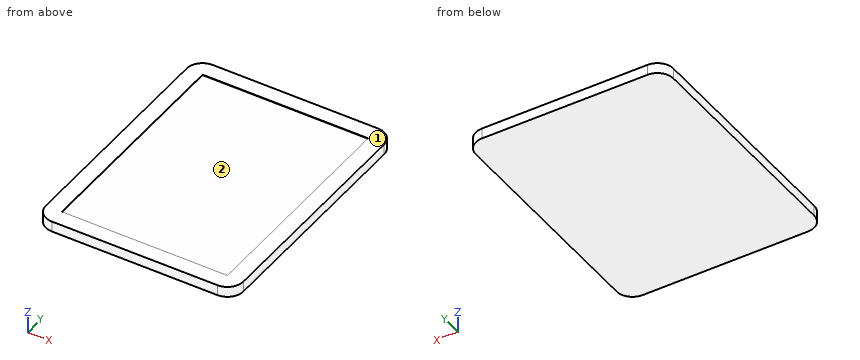
Autodesk Inventor part; units mm, degrees
ref_plane "YZ Plane" through (0, 0, 0) normal (1, 0, 0) x (0, 1, 0)
ref_plane "XZ Plane" through (0, 0, 0) normal (0, 1, 0) x (-1, 0, 0)
ref_plane "XY Plane" through (0, 0, 0) normal (0, 0, 1) x (1, 0, 0)
sketch "Skizze1" plane through (0, 0, 0) normal (0, 0, 1) x (1, 0, 0)
  line L0 (-93, 120.5) -> (93, 120.5)
  line L1 (93, 120.5) -> (93, -120.5)
  line L2 (93, -120.5) -> (-93, -120.5)
  line L3 (-93, -120.5) -> (-93, 120.5)
  line L4 (-130.2, 0) -> (130.2, 0)
  line L5 (0, -168.7) -> (0, 168.7)
  point P0 (0, 0)
  dimension "d0" = 241
  dimension "d1" = 186
extrude "Extrusion1" add sketch "Skizze1" along normal blind 10
sketch "Skizze3" plane through (0, 0, 10) normal (0, 0, 1) x (1, 0, 0)
  line L0 (93, 120.5) -> (93, -120.5)
  line L1 (-93, 120.5) -> (93, 120.5)
  line L2 (-93, -120.5) -> (-93, 120.5)
  line L3 (93, -120.5) -> (-93, -120.5)
  line L4 (78, 105.5) -> (78, -105.5)
  line L5 (78, -105.5) -> (-78, -105.5)
  line L6 (-78, -105.5) -> (-78, 105.5)
  line L7 (-78, 105.5) -> (78, 105.5)
  point P0 (0, 0)
  dimension "d5" = 15
extrude "Extrusion2" cut sketch "Skizze3" against normal blind 0.5 contours L4 L5 L6 L7
fillet "Rundung2" radius 15 4 edges at (-93, -120.5, 5) (93, -120.5, 5) (93, 120.5, 5) (-93, 120.5, 5)
properties part number "tablet"
The model under review builds one solid part; all positions refer to its coordinate system, in mm. Face numbers are marked on the shaded views. A direction names the side the tool comes from. Give positions to 0.01 mm unless a question says otherwise; leave off trailing zeros. Write each loop counter-clockwise with the first axis right and the second up, starting at its lowest first coordinate (ties: lowest second). Pieces come first, ordered by that corner, then holes. Notation, with made-up numbers: M 56,44.5 L 86,44.5 A11 cw 86,52.5 Z; hole C 37.25,-9.75 d9. An arc over 180 degrees is marked long. Answer in a Markdown table with one row per item.
Item 1: For P1, Ø5, axis at x = 5.5, y = 26.5, coming from the -Z side; P2, Ø10, axis at x = 49, y = 7, coming from the +Z side, all flat-tipped, find the tip position at first contact; note any pin that passes through.
Check sheet entries:
| item | result |
|---|---|
| P1 | z = 0 |
| P2 | z = 9.5 |
Item 2: Add section B-B on y = -23. Give the boundary of the cut face in (x, z).
Check sheet entries:
| item | result |
|---|---|
| outline | M -93,0 L 93,0 L 93,10 L 78,10 L 78,9.5 L -78,9.5 L -78,10 L -93,10 Z |
Item 3: Tool access review of the marked faces 1 and 2: name each direction out of +Z, -Z, +X, -X, +Y, -Y from which nothing blocks a thin tool from reaching the whole face with its end or side.
Check sheet entries:
| item | result |
|---|---|
| face 1 | +Z, +X, -X, +Y, -Y |
| face 2 | +Z |
Item 4: Add section A-A on x = -23. Give the boundary of the cut face in (y, z), plus the area to 3 significant figures.
Check sheet entries:
| item | result |
|---|---|
| outline | M -120.5,0 L 120.5,0 L 120.5,10 L 105.5,10 L 105.5,9.5 L -105.5,9.5 L -105.5,10 L -120.5,10 Z |
| area | 2,300 mm2 |
Item 5: For line 1 along Y through (x, z) = (57, 9.75); line 2 along Z through (x, y) = (21, -51); line 3 along X through (y, z) = (-111, 8), list the stretches that pass through material, from the lowest coordinate up.
Check sheet entries:
| item | result |
|---|---|
| line 1 | -120.5 to -105.5, 105.5 to 120.5 |
| line 2 | 0 to 9.5 |
| line 3 | -91.96 to 91.96 |
